```python
from build123d import *

# Parameters (mm, degrees)
SALIENTE_EXTRUIR1_DEPTH = 3
CROQUIS4_R              = 1.5
CROQUIS4_W              = 15
CROQUIS4_H              = 3.2
CROQUIS4_H_2            = 3
CORTAR_EXTRUIR1_DEPTH   = 3
SALIENTE_EXTRUIR2_DEPTH = 3
REDONDEO1_R             = 1
REDONDEO2_R             = 0.25
CROQUIS6_R              = 1.5
CROQUIS6_W              = 13
CROQUIS6_H              = 7
CORTAR_EXTRUIR2_DEPTH   = 5


with BuildPart() as part:
    # Croquis3 → Saliente-Extruir1 (new body)
    with BuildSketch(Plane(origin=(0, 0, 0), x_dir=(1, 0, 0), z_dir=(0, 1, 0))):
        with BuildLine():
            Line((-50, -40), (50, -40))
            Line((50, -40), (50, -35.05))
            Line((50, -35.05), (53, -35.05))
            Line((53, -35.05), (53, -30.05))
            Line((53, -30.05), (56.1, -30.05))
            Line((56.1, -30.05), (56.1, -35.05))
            Line((56.1, -35.05), (58.1, -35.05))
            Line((58.1, -35.05), (58.1, -27.55))
            ThreePointArc((58.1, -27.55), (57.367766953, -25.782233047), (55.6, -25.05))
            Line((55.6, -25.05), (50, -25.05))
            Line((50, -25.05), (50, 38.139923373))
            ThreePointArc((50, 38.139923373), (49.505732321, 39.632249697), (48.218369714, 40.534489086))
            Line((48.218369714, 40.534489086), (0.718369714, 54.784489086))
            ThreePointArc((0.718369714, 54.784489086), (0, 54.889923373), (-0.718369714, 54.784489086))
            Line((-0.718369714, 54.784489086), (-48.218369714, 40.534489086))
            ThreePointArc((-48.218369714, 40.534489086), (-49.505732321, 39.632249697), (-50, 38.139923373))
            Line((-50, 38.139923373), (-50, -25.05))
            Line((-50, -25.05), (-55.6, -25.05))
            ThreePointArc((-55.6, -25.05), (-57.367766953, -25.782233047), (-58.1, -27.55))
            Line((-58.1, -27.55), (-58.1, -35.05))
            Line((-58.1, -35.05), (-56.1, -35.05))
            Line((-56.1, -35.05), (-56.1, -30.05))
            Line((-56.1, -30.05), (-53, -30.05))
            Line((-53, -30.05), (-53, -35.05))
            Line((-53, -35.05), (-50, -35.05))
            Line((-50, -35.05), (-50, -40))
        make_face()
        Polygon((-31.156326057, 42.52101023), (-16.056326057, 47.05101023), (-15.165547612, 44.081748746), (-30.265547612, 39.551748746), align=None, mode=Mode.SUBTRACT)
        Polygon((15.165547612, 44.081748746), (30.265547612, 39.551748746), (31.156326057, 42.52101023), (16.056326057, 47.05101023), align=None, mode=Mode.SUBTRACT)
    extrude(amount=SALIENTE_EXTRUIR1_DEPTH)

    # Croquis4 → Cortar-Extruir1 (cut, symmetric)
    with BuildSketch(Plane(origin=(0, 3, 0), x_dir=(1, 0, 0), z_dir=(0, 1, 0))):
        with Locations(Location((32.75, 24, 0), (0, 0, 270))):
            Circle(CROQUIS4_R)
        with Locations(Location((-32.736745283, 24, 0), (0, 0, 270))):
            Circle(CROQUIS4_R)
        with Locations(Location((32.75, -24, 0), (0, 0, 270))):
            Circle(CROQUIS4_R)
        with Locations(Location((-32.736745283, -24, 0), (0, 0, 270))):
            Circle(CROQUIS4_R)
        with Locations((-30.5, -38.4)):
            Rectangle(CROQUIS4_W, CROQUIS4_H)
        with Locations((30.5, -38.4)):
            Rectangle(CROQUIS4_W, CROQUIS4_H)
        with Locations((0, -35.3)):
            Rectangle(CROQUIS4_W, CROQUIS4_H_2)
        with BuildLine():
            Line((-40.069692956, 26.698449706), (-40.069692956, 21.030308718))
            ThreePointArc((-40.069692956, 21.030308718), (-41.260824034, 19.839177641), (-42.451955111, 21.030308718))
            Line((-42.451955111, 21.030308718), (-42.451955111, 26.698449706))
            ThreePointArc((-42.451955111, 26.698449706), (-41.260824034, 27.889580784), (-40.069692956, 26.698449706))
        make_face()
    extrude(amount=CORTAR_EXTRUIR1_DEPTH, both=True, mode=Mode.SUBTRACT)

    # Croquis5 → Saliente-Extruir2 (add)
    with BuildSketch(Plane(origin=(0, 0, 0), x_dir=(1, 0, 0), z_dir=(0, 1, 0))):
        with BuildLine():
            Line((-50, -40), (49.999265674, -40))
            Line((49.999265674, -40), (49.999265674, -40.5))
            ThreePointArc((49.999265674, -40.5), (49.267032626, -42.267766953), (47.499265674, -43))
            Line((47.499265674, -43), (-47.5, -43))
            ThreePointArc((-47.5, -43), (-49.267766953, -42.267766953), (-50, -40.5))
            Line((-50, -40.5), (-50, -40))
        make_face()
    extrude(amount=SALIENTE_EXTRUIR2_DEPTH)

    # Redondeo1
    redondeo1_edges = [part.edges().sort_by_distance(p)[0] for p in [
        (-50, 1.5, 35.05),
        (-58.1, 1.5, 35.05),
        (-50, 1.5, 25.05),
        (50, 1.5, 25.05),
        (58.1, 1.5, 35.05),
        (50, 1.5, 35.05),
    ]]
    fillet(redondeo1_edges, radius=REDONDEO1_R)

    # Redondeo2
    redondeo2_edges = [part.edges().sort_by_distance(p)[0] for p in [
        (-53, 1.5, 35.05),
        (-53, 1.5, 30.05),
        (-56.1, 1.5, 30.05),
        (-56.1, 1.5, 35.05),
        (56.1, 1.5, 35.05),
        (56.1, 1.5, 30.05),
        (53, 1.5, 30.05),
        (53, 1.5, 35.05),
    ]]
    fillet(redondeo2_edges, radius=REDONDEO2_R)

    # Croquis6 → Cortar-Extruir2 (cut, symmetric)
    with BuildSketch(Plane(origin=(0, 3, 0), x_dir=(1, 0, 0), z_dir=(0, 1, 0))):
        with Locations(Location((-35.361176909, 27.833892011, 0), (0, 0, 270))):
            Circle(CROQUIS6_R)
        with Locations(Location((34.977904809, 27.833892011, 0), (0, 0, 270))):
            Circle(CROQUIS6_R)
        with Locations(Location((34.977904809, -28.23447772, 0), (0, 0, 270))):
            Circle(CROQUIS6_R)
        with Locations(Location((-35.361176909, -28.23447772, 0), (0, 0, 270))):
            Circle(CROQUIS6_R)
        with Locations((0, 36.081396556)):
            Rectangle(CROQUIS6_W, CROQUIS6_H)
    extrude(amount=CORTAR_EXTRUIR2_DEPTH, both=True, mode=Mode.SUBTRACT)


solid = part.part
```
The listing builds one solid part. Answer for the finished solid, in the listing's coordinates (mm). A direction names the side the tool comes from. Round coordinates to 2 decimals unless told otherwise and drop trailing zeros. Order: outer loops, then holes, each group sorted by start corner. A loop starts at its lowest first (then second) coordinate and runs counter-clockwise, first axis right, second up. Notation, with made-up numbers: (13.25, -35) - (46.25, -35) arc R22 cw to (46.25, -27) - close; hole circle Ø6 at (66.25, 83.25). An arc over 180 degrees is marked (long way). Put each result on its own line as item: value. Start each with the question number.
(1) Find section A-A (x = -20). Give the vertices of the cut face in (y, z), plus the area to 3 significant figures.
(2) Find section B-B (z = -24). Give the vertices of the cut face in (x, y).
(3) For faces 1 (the cylindrical face through (57.387, 1.479, 25.802)), 2 (the cylindrical face through (-49.248, 1.479, 42.287)), 3 (the flat face through (30.7, 1.5, -41)), 4 (the flat face through (55, 1, 30.05)), 5 (the flat face through (-53, 1, 25.05)), determine the directions among +Z, -Z, +X, -X, +Y, -Y from which every point of the face is accessible in a straight line to the end or side of a thin tool.
(4) Given P1, Ø0.9, axis at y = 1.5, z = -2, coming from the +X side; P2, Ø0.9, axis at y = 1, z = -23, coming from the -X side; P3, Ø1.5, axis at y = 1.5, z = 35.5, coming from the +X side, each flat-ended and moving along its own axis, determine where each tip first touches the part or whether it passes through.
(5) Find section D-D (x = 42.5). Give the vertices of the cut face in (y, z).
(6) Find section C-C (y = 2). State how many separate pieces and enclosed holes the cut face has, plus the area to 3 significant figures.
(7) Straight lines are drawn through the part: probe 1 along X at (y, z) = (1.75, 24); probe 2 along X at (y, z) = (1.85, -24); probe 3 along X at (y, z) = (1.8, -26). For each, find the intervals that lie inside material, in ascending order. Write a range as from..to.
(8) Determine the mould class of faces 6 (the flat face through (56.1, 1, 33)), 7 (the cylindrical face through (-34.911, 1.521, 29.665)), 8 (the flat face through (-24.14, 1.48, -47.76)) for opening direction Z: released by +Z, released by -Z, zero draft, split by the parting line, or undercut.
Reply:
1. outline: (0, -49) - (3, -49) - (3, -45.87) - (0, -45.87) - close; (0, -42.63) - (3, -42.63) - (3, 43) - (0, 43) - close
1. area: 266 mm^2
2. outline: (-50, 0) - (-42.45, 0) - (-42.45, 3) - (-50, 3) - close; (-40.07, 0) - (-34.24, 0) - (-34.24, 3) - (-40.07, 3) - close; (-31.24, 0) - (31.25, 0) - (31.25, 3) - (-31.24, 3) - close; (34.25, 0) - (50, 0) - (50, 3) - (34.25, 3) - close
3. face 1: -Z, +X, +Y, -Y
3. face 2: +Z, -X, +Y, -Y
3. face 3: +Y, -Y
3. face 4: +Z, +Y, -Y
3. face 5: -Z, -X, +Y, -Y
4. P1: x = 50
4. P2: x = -50
4. P3: x = 57.81
5. outline: (0, -42.25) - (3, -42.25) - (3, 43) - (0, 43) - close
6. separate pieces: 1
6. enclosed holes: 15
6. area: 8,770 mm^2
7. probe 1: -50..-34.24, -31.24..31.25, 34.25..50
7. probe 2: -50..-42.45, -40.07..-34.24, -31.24..31.25, 34.25..50
7. probe 3: -50..-42.45, -40.07..50
8. face 6: zero draft
8. face 7: undercut
8. face 8: released by -Z
